from build123d import *

# Parameters (mm, degrees)
SKETCH_1_R          = 2.5
SKETCH_1_R_2        = 1.5
EXTRUDE_1_DEPTH     = 10
FILLET_1_R          = 0.2
CUT_EXTRUDE_1_DEPTH = 10


with BuildPart() as part:
    # Эскиз1 → Вытянуть1 (new body)
    with BuildSketch(Plane.XY):
        with BuildLine():
            Line((-0.685932761, 9.95), (0, 9.95))
            Line((0, 9.95), (0.676, 9.95))
            Line((0.676, 9.95), (1.110862137, 11.144773901))
            ThreePointArc((1.110862137, 11.144773901), (2.487539236, 10.920263209), (3.825633205, 10.526373097))
            Line((3.825633205, 10.526373097), (3.699139141, 9.262255307))
            Line((3.699139141, 9.262255307), (4.317143204, 8.964640236))
            Line((4.317143204, 8.964640236), (4.926198159, 8.671334828))
            Line((4.926198159, 8.671334828), (5.836388374, 9.559109307))
            ThreePointArc((5.836388374, 9.559109307), (6.979320043, 8.759514355), (8.013998536, 7.824054413))
            Line((8.013998536, 7.824054413), (7.351551169, 6.740007356))
            Line((7.351551169, 6.740007356), (7.779223251, 6.203723528))
            Line((7.779223251, 6.203723528), (8.200702357, 5.675205446))
            Line((8.200702357, 5.675205446), (9.405946315, 6.08014588))
            ThreePointArc((9.405946315, 6.08014588), (10.088760919, 4.863836255), (10.615093172, 3.572085797))
            Line((10.615093172, 3.572085797), (9.547898328, 2.882818288))
            Line((9.547898328, 2.882818288), (9.700532726, 2.214083293))
            Line((9.700532726, 2.214083293), (9.850956878, 1.555032024))
            Line((9.850956878, 1.555032024), (11.112541232, 1.396934994))
            ThreePointArc((11.112541232, 1.396934994), (11.199998965, 0.004815734), (11.11373842, -1.38737822))
            Line((11.11373842, -1.38737822), (9.853167125, -1.545348298))
            Line((9.853167125, -1.545348298), (9.700532726, -2.214083293))
            Line((9.700532726, -2.214083293), (9.550108575, -2.873134562))
            Line((9.550108575, -2.873134562), (10.618161071, -3.562956001))
            ThreePointArc((10.618161071, -3.562956001), (10.092939856, -4.855158602), (9.411171473, -6.072054966))
            Line((9.411171473, -6.072054966), (8.206895332, -5.667439701))
            Line((8.206895332, -5.667439701), (7.779223251, -6.203723528))
            Line((7.779223251, -6.203723528), (7.357744145, -6.732241611))
            Line((7.357744145, -6.732241611), (8.020723888, -7.817159863))
            ThreePointArc((8.020723888, -7.817159863), (6.986850228, -8.753509233), (5.844606595, -9.554086756))
            Line((5.844606595, -9.554086756), (4.935147268, -8.667025164))
            Line((4.935147268, -8.667025164), (4.317143204, -8.964640236))
            Line((4.317143204, -8.964640236), (3.70808825, -9.257945643))
            Line((3.70808825, -9.257945643), (3.83468397, -10.523079343))
            ThreePointArc((3.83468397, -10.523079343), (2.496929223, -10.918120005), (1.120445701, -11.143814492))
            Line((1.120445701, -11.143814492), (0.685932761, -9.95))
            Line((0.685932761, -9.95), (0, -9.95))
            Line((0, -9.95), (-0.676, -9.95))
            Line((-0.676, -9.95), (-1.110862137, -11.144773901))
            ThreePointArc((-1.110862137, -11.144773901), (-2.487539236, -10.920263209), (-3.825633205, -10.526373097))
            Line((-3.825633205, -10.526373097), (-3.699139141, -9.262255307))
            Line((-3.699139141, -9.262255307), (-4.317143204, -8.964640236))
            Line((-4.317143204, -8.964640236), (-4.926198159, -8.671334828))
            Line((-4.926198159, -8.671334828), (-5.836388374, -9.559109307))
            ThreePointArc((-5.836388374, -9.559109307), (-6.979320043, -8.759514355), (-8.013998536, -7.824054413))
            Line((-8.013998536, -7.824054413), (-7.351551169, -6.740007356))
            Line((-7.351551169, -6.740007356), (-7.779223251, -6.203723528))
            Line((-7.779223251, -6.203723528), (-8.200702357, -5.675205446))
            Line((-8.200702357, -5.675205446), (-9.405946315, -6.08014588))
            ThreePointArc((-9.405946315, -6.08014588), (-10.088760919, -4.863836255), (-10.615093172, -3.572085797))
            Line((-10.615093172, -3.572085797), (-9.547898328, -2.882818288))
            Line((-9.547898328, -2.882818288), (-9.700532726, -2.214083293))
            Line((-9.700532726, -2.214083293), (-9.850956878, -1.555032024))
            Line((-9.850956878, -1.555032024), (-11.112541232, -1.396934994))
            ThreePointArc((-11.112541232, -1.396934994), (-11.199998965, -0.004815734), (-11.11373842, 1.38737822))
            Line((-11.11373842, 1.38737822), (-9.853167125, 1.545348298))
            Line((-9.853167125, 1.545348298), (-9.700532726, 2.214083293))
            Line((-9.700532726, 2.214083293), (-9.550108575, 2.873134562))
            Line((-9.550108575, 2.873134562), (-10.618161071, 3.562956001))
            ThreePointArc((-10.618161071, 3.562956001), (-10.092939856, 4.855158602), (-9.411171473, 6.072054966))
            Line((-9.411171473, 6.072054966), (-8.206895332, 5.667439701))
            Line((-8.206895332, 5.667439701), (-7.779223251, 6.203723528))
            Line((-7.779223251, 6.203723528), (-7.357744145, 6.732241611))
            Line((-7.357744145, 6.732241611), (-8.020723888, 7.817159863))
            ThreePointArc((-8.020723888, 7.817159863), (-6.986850228, 8.753509233), (-5.844606595, 9.554086756))
            Line((-5.844606595, 9.554086756), (-4.935147268, 8.667025164))
            Line((-4.935147268, 8.667025164), (-4.317143204, 8.964640236))
            Line((-4.317143204, 8.964640236), (-3.70808825, 9.257945643))
            Line((-3.70808825, 9.257945643), (-3.83468397, 10.523079343))
            ThreePointArc((-3.83468397, 10.523079343), (-2.496929223, 10.918120005), (-1.120445701, 11.143814492))
            Line((-1.120445701, 11.143814492), (-0.685932761, 9.95))
        make_face()
        Circle(SKETCH_1_R, mode=Mode.SUBTRACT)
        with Locations((0, 6)):
            Circle(SKETCH_1_R_2, mode=Mode.SUBTRACT)
        with Locations((0, -6)):
            Circle(SKETCH_1_R_2, mode=Mode.SUBTRACT)
    extrude(amount=EXTRUDE_1_DEPTH)

    # Скругление1
    fillet_1_edges = [part.edges().sort_by_distance(p)[0] for p in [
        (9.547898328, 2.882818288, 5),
        (9.850956878, 1.555032024, 5),
        (11.112541232, 1.396934994, 5),
        (11.11373842, -1.38737822, 5),
        (9.853167125, -1.545348298, 5),
        (9.550108575, -2.873134562, 5),
        (10.618161071, -3.562956001, 5),
        (9.411171473, -6.072054966, 5),
        (8.206895332, -5.667439701, 5),
        (7.357744145, -6.732241611, 5),
        (8.020723888, -7.817159863, 5),
        (5.844606595, -9.554086756, 5),
        (4.935147268, -8.667025164, 5),
        (3.70808825, -9.257945643, 5),
        (3.83468397, -10.523079343, 5),
        (1.120445701, -11.143814492, 5),
        (0.685932761, -9.95, 5),
        (-0.676, -9.95, 5),
        (-1.110862137, -11.144773901, 5),
        (-3.825633205, -10.526373097, 5),
        (-3.699139141, -9.262255307, 5),
        (-4.926198159, -8.671334828, 5),
        (-5.836388374, -9.559109307, 5),
        (-8.013998536, -7.824054413, 5),
        (-7.351551169, -6.740007356, 5),
        (-8.200702357, -5.675205446, 5),
        (-9.405946315, -6.08014588, 5),
        (-10.615093172, -3.572085797, 5),
        (-9.547898328, -2.882818288, 5),
        (-9.850956878, -1.555032024, 5),
        (-11.112541232, -1.396934994, 5),
        (-11.11373842, 1.38737822, 5),
        (-9.853167125, 1.545348298, 5),
        (-10.618161071, 3.562956001, 5),
        (-9.411171473, 6.072054966, 5),
        (-8.206895332, 5.667439701, 5),
        (-7.357744145, 6.732241611, 5),
        (-8.020723888, 7.817159863, 5),
        (-5.844606595, 9.554086756, 5),
        (-4.935147268, 8.667025164, 5),
        (-3.70808825, 9.257945643, 5),
        (-3.83468397, 10.523079343, 5),
        (-1.120445701, 11.143814492, 5),
        (-0.685932761, 9.95, 5),
        (0.676, 9.95, 5),
        (1.110862137, 11.144773901, 5),
        (3.825633205, 10.526373097, 5),
        (3.699139141, 9.262255307, 5),
        (4.926198159, 8.671334828, 5),
        (5.836388374, 9.559109307, 5),
        (8.013998536, 7.824054413, 5),
        (7.351551169, 6.740007356, 5),
        (8.200702357, 5.675205446, 5),
        (9.405946315, 6.08014588, 5),
        (10.615093172, 3.572085797, 5),
    ]]
    fillet(fillet_1_edges, radius=FILLET_1_R)

    # Эскиз2 → Вырез-Вытянуть1 (cut)
    with BuildSketch(Plane.XY.offset(10)):
        with BuildLine():
            Line((4.740104239, 12.147692744), (6.542041974, 11.279925266))
            Line((6.542041974, 11.279925266), (5.524607217, 9.167200224))
            ThreePointArc((5.524607217, 9.167200224), (4.18975461, 8.700115095), (3.722669482, 10.034967702))
            Line((3.722669482, 10.034967702), (4.740104239, 12.147692744))
        make_face()
        with BuildLine():
            Line((-1, 13.00134713), (1, 13.00134713))
            Line((1, 13.00134713), (1, 10.656399244))
            ThreePointArc((1, 10.656399244), (0, 9.656399244), (-1, 10.656399244))
            Line((-1, 10.656399244), (-1, 13.00134713))
        make_face()
        with BuildLine():
            Line((9.541372699, 8.888038829), (10.788352303, 7.324375864))
            Line((10.788352303, 7.324375864), (8.95499822, 5.862324771))
            ThreePointArc((8.95499822, 5.862324771), (7.549676936, 6.020666451), (7.708018617, 7.425987736))
            Line((7.708018617, 7.425987736), (9.541372699, 8.888038829))
        make_face()
        with BuildLine():
            Line((12.45285528, 3.867999818), (12.897897147, 1.918143994))
            Line((12.897897147, 1.918143994), (10.611742, 1.396344))
            ThreePointArc((10.611742, 1.396344), (9.414293154, 2.148750978), (10.166700132, 3.346199825))
            Line((10.166700132, 3.346199825), (12.45285528, 3.867999818))
        make_face()
        with BuildLine():
            Line((12.897897147, -1.918143994), (12.45285528, -3.867999818))
            Line((12.45285528, -3.867999818), (10.166700132, -3.346199825))
            ThreePointArc((10.166700132, -3.346199825), (9.414293154, -2.148750978), (10.611742, -1.396344))
            Line((10.611742, -1.396344), (12.897897147, -1.918143994))
        make_face()
        with BuildLine():
            Line((10.788352303, -7.324375864), (9.541372699, -8.888038829))
            Line((9.541372699, -8.888038829), (7.708018617, -7.425987736))
            ThreePointArc((7.708018617, -7.425987736), (7.549676936, -6.020666451), (8.95499822, -5.862324771))
            Line((8.95499822, -5.862324771), (10.788352303, -7.324375864))
        make_face()
        with BuildLine():
            Line((6.542041974, -11.279925266), (4.740104239, -12.147692744))
            Line((4.740104239, -12.147692744), (3.722669482, -10.034967702))
            ThreePointArc((3.722669482, -10.034967702), (4.18975461, -8.700115095), (5.524607217, -9.167200224))
            Line((5.524607217, -9.167200224), (6.542041974, -11.279925266))
        make_face()
        with BuildLine():
            Line((1, -13.00134713), (-1, -13.00134713))
            Line((-1, -13.00134713), (-1, -10.656399244))
            ThreePointArc((-1, -10.656399244), (0, -9.656399244), (1, -10.656399244))
            Line((1, -10.656399244), (1, -13.00134713))
        make_face()
        with BuildLine():
            Line((-4.740104239, -12.147692744), (-6.542041974, -11.279925266))
            Line((-6.542041974, -11.279925266), (-5.524607217, -9.167200224))
            ThreePointArc((-5.524607217, -9.167200224), (-4.18975461, -8.700115095), (-3.722669482, -10.034967702))
            Line((-3.722669482, -10.034967702), (-4.740104239, -12.147692744))
        make_face()
        with BuildLine():
            Line((-9.541372699, -8.888038829), (-10.788352303, -7.324375864))
            Line((-10.788352303, -7.324375864), (-8.95499822, -5.862324771))
            ThreePointArc((-8.95499822, -5.862324771), (-7.549676936, -6.020666451), (-7.708018617, -7.425987736))
            Line((-7.708018617, -7.425987736), (-9.541372699, -8.888038829))
        make_face()
        with BuildLine():
            Line((-12.452855279, -3.867999818), (-12.897897147, -1.918143994))
            Line((-12.897897147, -1.918143994), (-10.611742, -1.396344))
            ThreePointArc((-10.611742, -1.396344), (-9.414293154, -2.148750978), (-10.166700132, -3.346199825))
            Line((-10.166700132, -3.346199825), (-12.452855279, -3.867999818))
        make_face()
        with BuildLine():
            Line((-12.897897147, 1.918143994), (-12.45285528, 3.867999818))
            Line((-12.45285528, 3.867999818), (-10.166700132, 3.346199825))
            ThreePointArc((-10.166700132, 3.346199825), (-9.414293154, 2.148750978), (-10.611742, 1.396344))
            Line((-10.611742, 1.396344), (-12.897897147, 1.918143994))
        make_face()
        with BuildLine():
            Line((-10.788352303, 7.324375864), (-9.541372699, 8.888038829))
            Line((-9.541372699, 8.888038829), (-7.708018617, 7.425987736))
            ThreePointArc((-7.708018617, 7.425987736), (-7.549676936, 6.020666451), (-8.95499822, 5.862324771))
            Line((-8.95499822, 5.862324771), (-10.788352303, 7.324375864))
        make_face()
        with BuildLine():
            Line((-6.542041974, 11.279925266), (-4.740104239, 12.147692744))
            Line((-4.740104239, 12.147692744), (-3.722669482, 10.034967702))
            ThreePointArc((-3.722669482, 10.034967702), (-4.18975461, 8.700115095), (-5.524607217, 9.167200224))
            Line((-5.524607217, 9.167200224), (-6.542041974, 11.279925266))
        make_face()
    extrude(amount=-CUT_EXTRUDE_1_DEPTH, mode=Mode.SUBTRACT)


solid = part.part
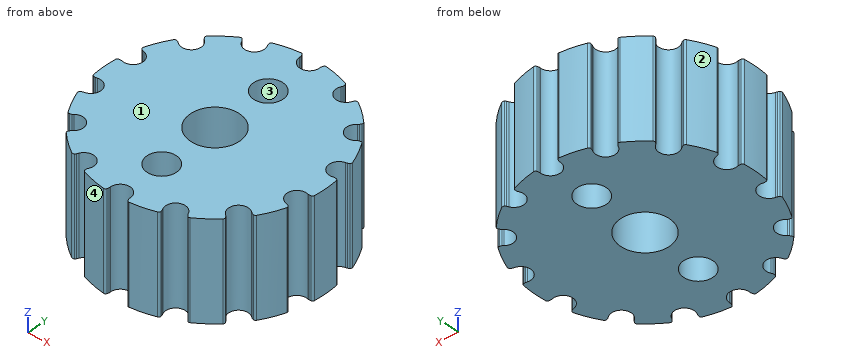
The listing builds one solid part. Answer for the finished solid, in the listing's coordinates (mm). Face numbers are marked on the shaded views. Give positions to 0.01 mm unless a question says otherwise; leave off trailing zeros. Loops run counter-clockwise (first coordinate to the right, second up) from the corner with the lowest first, then second, coordinate; pieces in that order, holes last. Notation, with made-up numbers: (-37.5, -28.75) - (-25.5, -28.75) arc R26 ccw to (-25.5, 3.25) - close; hole circle Ø9 at (3.25, 38.5). An arc over 180 degrees is marked (long way). Use one line per item in the form item = value.
1. Section C-C on y = 7 is taken. Give the vertices of the cut face in (x, z).
Calculated:
outline = (-7.4, 0) - (-1.12, 0) - (-1.12, 10) - (-7.4, 10) - close; (1.12, 0) - (7.4, 0) - (7.4, 10) - (1.12, 10) - close
2. Section D-D on z = 5 is taken. Count the separate pieces of the cut face and the enclosed holes in it, then the cut area to 3 significant figures.
Calculated:
separate_pieces = 1
enclosed_holes = 3
area = 323 mm^2
3. Given pin 1 Ø3 at (x, z) = (2, 5.5) entering from -Y; pin 2 Ø1.5 at (x, z) = (3, 6.5) entering from -Y; pin 3 Ø5 at (y, z) = (5.5, 3.5) entering from -X, each flat-ended and moving along its own axis, determine where each tip first touches the part or whether it passes through.
Calculated:
pin_1 = -11.13
pin_2 = -10.97
pin_3 = -10.58
4. The mould has two halves that part along Y. Classify the marked faces 1, 2, 3 and 4: pulls with the +Y half, pulls with the -Y half, needs draft (parallel to the pull), parting line crosses it, or undercut.
Calculated:
face_1 = needs draft
face_2 = pulls with the +Y half
face_3 = undercut
face_4 = pulls with the -Y half
5. Section A-A on x = 0 is taken. Give the vertices of the cut face in (y, z), then the cut area to 3 significant figures.
Calculated:
outline = (-9.66, 0) - (-7.5, 0) - (-7.5, 10) - (-9.66, 10) - close; (-4.5, 0) - (-2.5, 0) - (-2.5, 10) - (-4.5, 10) - close; (2.5, 0) - (4.5, 0) - (4.5, 10) - (2.5, 10) - close; (7.5, 0) - (9.66, 0) - (9.66, 10) - (7.5, 10) - close
area = 83.1 mm^2
6. Find the intervals of material crossed by line 1 along Y through (x, z) = (0, 4); line 2 along X through (y, z) = (9, 2); line 3 along Y through (x, z) = (7.5, 4.5), in increasing order. Write a range as [from, to].
Calculated:
line_1 = [-9.66, -7.5], [-4.5, -2.5], [2.5, 4.5], [7.5, 9.66]
line_2 = [-6.67, -5.42], [-3.82, 3.82], [5.42, 6.67]
line_3 = [-8.32, -7.2], [-6.09, 6.09], [7.2, 8.32]
7. Section B-B on y = 0 is taken. Give the vertices of the cut face in (x, z).
Calculated:
outline = (-11.2, 0) - (-2.5, 0) - (-2.5, 10) - (-11.2, 10) - close; (2.5, 0) - (11.2, 0) - (11.2, 10) - (2.5, 10) - close
